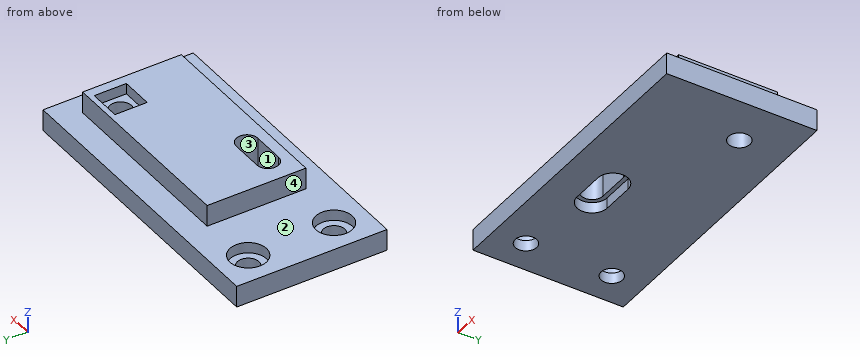
from build123d import *

# Parameters (mm, degrees)
ESQUISSE1_W             = 140
ESQUISSE1_H             = 70
ESQUISSE1_R             = 5
BOSS_EXTRU_1_DEPTH      = 10
ESQUISSE2_R             = 8.5
ENL_V_MAT_EXTRU_1_DEPTH = 5
ESQUISSE3_W             = 90
ESQUISSE3_H             = 46
BOSS_EXTRU_2_DEPTH      = 10
ESQUISSE4_R             = 5
ENL_V_MAT_EXTRU_2_DEPTH = 81.777472107
ESQUISSE5_W             = 15
ESQUISSE5_H             = 15
ENL_V_MAT_EXTRU_3_DEPTH = 5
ENL_V_MAT_EXTRU_4_DEPTH = 5


with BuildPart() as part:
    # Esquisse1 → Boss.-Extru.1 (new body)
    with BuildSketch(Plane.XY):
        Rectangle(ESQUISSE1_W, ESQUISSE1_H)
        with Locations((-55, 20)):
            Circle(ESQUISSE1_R, mode=Mode.SUBTRACT)
        with Locations((-55, -20)):
            Circle(ESQUISSE1_R, mode=Mode.SUBTRACT)
    extrude(amount=BOSS_EXTRU_1_DEPTH)

    # Esquisse2 → Enlèv. mat.-Extru.1 (cut)
    with BuildSketch(Plane.XY.offset(10)):
        with Locations((-55, 20)):
            Circle(ESQUISSE2_R)
        with Locations((-55, -20)):
            Circle(ESQUISSE2_R)
    extrude(amount=-ENL_V_MAT_EXTRU_1_DEPTH, mode=Mode.SUBTRACT)

    # Esquisse3 → Boss.-Extru.2 (add)
    with BuildSketch(Plane.XY.offset(10)):
        with Locations((15, 0)):
            Rectangle(ESQUISSE3_W, ESQUISSE3_H)
    extrude(amount=BOSS_EXTRU_2_DEPTH)

    # Esquisse4 → Enlèv. mat.-Extru.2 (cut, through all)
    with BuildSketch(Plane.XY.offset(20)):
        with Locations((48, 13)):
            Circle(ESQUISSE4_R)
        with BuildLine():
            Line((-18, -8), (-3, -8))
            ThreePointArc((-3, -8), (2, -13), (-3, -18))
            Line((-3, -18), (-18, -18))
            ThreePointArc((-18, -18), (-23, -13), (-18, -8))
        make_face()
    extrude(amount=-ENL_V_MAT_EXTRU_2_DEPTH, mode=Mode.SUBTRACT)

    # Esquisse5 → Enlèv. mat.-Extru.3 (cut)
    with BuildSketch(Plane.XY.offset(20)):
        with Locations((48, 13)):
            Rectangle(ESQUISSE5_W, ESQUISSE5_H)
    extrude(amount=-ENL_V_MAT_EXTRU_3_DEPTH, mode=Mode.SUBTRACT)

    # Esquisse6 → Enlèv. mat.-Extru.4 (cut)
    with BuildSketch(Plane(origin=(0, 0, 0), x_dir=(-1, 0, 0), z_dir=(0, 0, -1))):
        with BuildLine():
            Line((18, -20), (3, -20))
            ThreePointArc((3, -20), (-4, -13), (3, -6))
            Line((3, -6), (18, -6))
            ThreePointArc((18, -6), (25, -13), (18, -20))
        make_face()
    extrude(amount=-ENL_V_MAT_EXTRU_4_DEPTH, mode=Mode.SUBTRACT)


solid = part.part
Could you check a few things on this model? Use its own coordinates, in mm. Face numbers are marked on the shaded views. Give positions to 0.01 mm unless a question says otherwise; leave off trailing zeros. Order: outer loops, then holes, each group sorted by start corner. A loop starts at its lowest first (then second) coordinate and runs counter-clockwise, first axis right, second up. Notation, with made-up numbers: (-22, -16) - (-1, -16) arc R31 cw to (-1, 17) - close; hole circle Ø9 at (88, -16). An arc over 180 degrees is marked (long way). One line per item, written item: value. Start each with the question number.
1. Imagine slicing it at A-A on x = -11. List the corners of the cut face in (y, z) for me.
2. Imagine slicing it at C-C on z = 12.5. List the corners of the cut face in (x, y) for me.
3. Imagine slicing it at B-B on z = 2.75. List the corners of the cut face in (x, y) for me.
4. Imagine slicing it at D-D on y = 13. List the corners of the cut face in (x, z) for me.
5. For P1, Ø5, axis at y = 9.5, z = 16.5, coming from the -X side; P2, Ø7.5, axis at x = 50, y = 15, coming from the +Z side; P3, Ø2, axis at x = -40.5, y = -1.5, coming from the +Z side, each with a flat end and sliding along its axis, tell me the tip position at first contact or that it passes through.
6. Thinking about a two-plate mould opening in X: for the marked faces 1, 2, 3 and 4, which applies, +X half, -X half, draft (parallel to the pull), parting line (faces both ways), or undercut?
7. If I drill on probe 1 along Y at (x, z) = (-55, 8.4); probe 2 along Y at (x, z) = (-55, 1.2); probe 3 along X at (y, z) = (20, 19.25), over which ranges is the centre line in solid material (lowest first)?
Values:
1. outline: (-35, 0) - (-20, 0) - (-20, 5) - (-18, 5) - (-18, 20) - (-23, 20) - (-23, 10) - (-35, 10) - close; (-8, 5) - (-6, 5) - (-6, 0) - (35, 0) - (35, 10) - (23, 10) - (23, 20) - (-8, 20) - close
2. outline: (-30, -23) - (60, -23) - (60, 23) - (-30, 23) - close; hole (-18, -18) - (-3, -18) arc R5 ccw to (-3, -8) - (-18, -8) arc R5 ccw to start; hole circle Ø10 at (48, 13)
3. outline: (-70, -35) - (70, -35) - (70, 35) - (-70, 35) - close; hole circle Ø10 at (-55, -20); hole circle Ø10 at (-55, 20); hole (-18, -20) - (-3, -20) arc R7 ccw to (-3, -6) - (-18, -6) arc R7 ccw to start; hole circle Ø10 at (48, 13)
4. outline: (-70, 0) - (43, 0) - (43, 15) - (40.5, 15) - (40.5, 20) - (-30, 20) - (-30, 10) - (-50.18, 10) - (-50.18, 5) - (-59.82, 5) - (-59.82, 10) - (-70, 10) - close; (53, 0) - (70, 0) - (70, 10) - (60, 10) - (60, 20) - (55.5, 20) - (55.5, 15) - (53, 15) - close
5. P1: x = -30
5. P2: z = 15
5. P3: z = 10
6. face 1: undercut
6. face 2: draft
6. face 3: undercut
6. face 4: -X half
7. probe 1: -35 to -28.5, -11.5 to 11.5, 28.5 to 35
7. probe 2: -35 to -25, -15 to 15, 25 to 35
7. probe 3: -30 to 40.5, 55.5 to 60
